from build123d import *

# Parameters (mm, degrees)
F1_DEPTH = 0.3
F3_DEPTH = 30


with BuildPart() as f1:
    # F0 (on Top) → F1 (new body, symmetric)
    with BuildSketch(Plane.XY):
        Polygon((30, 9.5), (-30, 9.5), (-11, -9.5), (11, -9.5), align=None)
    extrude(amount=F1_DEPTH, both=True)

    # F2 (on Right) → F3 (cut, symmetric)
    with BuildSketch(Plane.YZ):
        Polygon((9.5, 0), (9.5, 0.3), (7.956634, 0.3), align=None)
        Polygon((9.5, -0.3), (9.5, 0), (7.956634, -0.3), align=None)
    extrude(amount=F3_DEPTH, both=True, mode=Mode.SUBTRACT)


solid = f1.part
Work out the finished part from the listing and answer in its coordinate system (mm). Coordinates: 2 decimals unless noted, no trailing zeros. Write each loop counter-clockwise with the first axis right and the second up, starting at its lowest first coordinate (ties: lowest second). Pieces come first, ordered by that corner, then holes. Notation, with made-up numbers: M 39,28 L 71,28 A11 ccw 71,44 Z; hole C -24,-13.75 d4. An arc over 180 degrees is marked long. Write item = value, one per line.
1. Straight lines are drawn through the part: line 1 (X direction, y = 0.5, z = 0.2); line 2 (X direction, y = 4, z = 0.15); line 3 (Z direction, x = 16, y = 8.75). For each, find the intervals that lie inside material, in ascending order. Write a range as from..to.
Solution:
line_1 = -21..21
line_2 = -24.5..24.5
line_3 = -0.15..0.15
2. The part is cut by section C-C (z = -0.15). Determine the outline of the cut face in (x, y), then the cut area to 3 significant figures.
Solution:
outline = M -29.23,8.73 L -11,-9.5 L 11,-9.5 L 29.23,8.73 Z
area = 733 mm2
3. The part is cut by section D-D (x = -23). Determine the outline of the cut face in (y, z), then the cut area to 3 significant figures.
Solution:
outline = M 2.5,-0.3 L 7.96,-0.3 L 9.5,0 L 7.96,0.3 L 2.5,0.3 Z
area = 3.74 mm2
4. The part is cut by section A-A (x = 20). Determine the outline of the cut face in (y, z).
Solution:
outline = M -0.5,-0.3 L 7.96,-0.3 L 9.5,0 L 7.96,0.3 L -0.5,0.3 Z
5. The part is cut by section B-B (y = -2.75). Determine the outline of the cut face in (x, z), then the cut area to 3 significant figures.
Solution:
outline = M -17.75,-0.3 L 17.75,-0.3 L 17.75,0.3 L -17.75,0.3 Z
area = 21.3 mm2
